from build123d import *

# Parameters (mm, degrees)
IZIM1_W                     = 110
IZIM1_H                     = 80.4
Y_KSEKLIK_EKSTR_ZYON1_DEPTH = 40
KES_EKSTR_ZYON1_DEPTH       = 30
KES_EKSTR_ZYON2_DEPTH       = 106.305080599


with BuildPart() as part:
    # Çizim1 → Yükseklik-Ekstrüzyon1 (new body)
    with BuildSketch(Plane.XY):
        Rectangle(IZIM1_W, IZIM1_H)
    extrude(amount=Y_KSEKLIK_EKSTR_ZYON1_DEPTH)

    # Çizim2 → Kes-Ekstrüzyon1 (cut)
    with BuildSketch(Plane.XY.offset(40)):
        Polygon((30.097607873, 15.947775896), (-10.133916247, 15.947775896), (-10.133916247, -26.710477825), (9.889023344, -26.710477825), (9.889023344, -23.599429186), (30.097607873, -23.599429186), align=None)
    extrude(amount=-KES_EKSTR_ZYON1_DEPTH, mode=Mode.SUBTRACT)

    # Çizim3 → Kes-Ekstrüzyon2 (cut, through all)
    with BuildSketch(Plane(origin=(0, 40.2, 0), x_dir=(1, 0, 0), z_dir=(0, 1, 0))):
        Polygon((9.889023344, -40), (10, -15), (-10, -15), (-10, -40), align=None)
    extrude(amount=-KES_EKSTR_ZYON2_DEPTH, mode=Mode.SUBTRACT)


solid = part.part
Source: CAD feature listing. Evaluate the final solid. Frame: model axes, mm. A direction names the side the tool comes from. Round coordinates to 2 decimals unless told otherwise and drop trailing zeros. Loops run counter-clockwise (first coordinate to the right, second up) from the corner with the lowest first, then second, coordinate; pieces in that order, holes last. Notation, with made-up numbers: M 24.5,12.5 L 39.5,12.5 A31 ccw 39.5,45.5 Z; hole C 0.5,4 d1. An arc over 180 degrees is marked long. Return JSON: item names as keys, results as strings. Group by question number.
1. Section query C-C on x = 16.5. Output: boundary loops of the cut face in (y, z).
2. Section query A-A on z = 37. Output: boundary loops of the cut face in (x, y).
3. Pin query (flat end, axial travel): pin 1 (5 mm diameter, centred on x = 4, y = 31, fed in from -Z); pin 2 (10 mm diameter, centred on x = 2, y = 30.5, fed in from +Z); pin 3 (12 mm diameter, centred on x = 10, y = -6, fed in from +Z). Return the tip coordinate at first contact, or that it passes through.
4. Section query D-D on z = 23. Output: boundary loops of the cut face in (x, y), and give its area (3 significant figures).
5. Reachability of faces 1 (the face through (30.098, -4, 25)), 2 (the face through (37, 1, 40)), 3 (the face through (-10, 28, 27)) from +Z, -Z, +X, -X, +Y, -Y: full face, straight path, thin tool, end or side. Return the list, or none.
6. Section query B-B on y = -30.5. Output: boundary loops of the cut face in (x, z).
7. Material intervals for line 1 along X through (y, z) = (-5, 24.5); line 2 along X through (y, z) = (-36, 17); line 3 along Y through (x, z) = (10.5, 35.5), sorted ascending. Write a range as from..to.
Checks:
{
 "1": {"outline": "M -40.2,0 L 40.2,0 L 40.2,40 L 15.95,40 L 15.95,10 L -23.6,10 L -23.6,40 L -40.2,40 Z"},
 "2": {"outline": "M -55,-40.2 L -10,-40.2 L -10,-26.71 L -10.13,-26.71 L -10.13,15.95 L -10,15.95 L -10,40.2 L -55,40.2 Z; M 9.9,-40.2 L 55,-40.2 L 55,40.2 L 9.9,40.2 L 9.9,15.95 L 30.1,15.95 L 30.1,-23.6 L 9.9,-23.6 Z"},
 "3": {"pin 1": "stops at z = 0", "pin 2": "stops at z = 15", "pin 3": "stops at z = 10"},
 "4": {"outline": "M -55,-40.2 L -10,-40.2 L -10,-26.71 L -10.13,-26.71 L -10.13,15.95 L -10,15.95 L -10,40.2 L -55,40.2 Z; M 9.96,-40.2 L 55,-40.2 L 55,40.2 L 9.96,40.2 L 9.96,15.95 L 30.1,15.95 L 30.1,-23.6 L 9.96,-23.6 Z", "area": "6,440 mm²"},
 "5": {"face 1": "+Z", "face 2": "+Z, +X, -X, +Y, -Y", "face 3": "+Z, +Y, -Y"},
 "6": {"outline": "M -55,0 L 55,0 L 55,40 L 9.89,40 L 10,15 L -10,15 L -10,40 L -55,40 Z"},
 "7": {"line 1": "x = -55..-10.13, 30.1..55", "line 2": "x = -55..-10, 9.99..55", "line 3": "y = -40.2..-23.6, 15.95..40.2"}
}
